```python
from build123d import *

# Parameters (mm, degrees)
BOSS_EXTRU_1_DEPTH           = 7.5
R_P_TITION_CIRCULAIRE1_COUNT = 33
ENL_V_MAT_EXTRU_3_DEPTH      = 129.364948487
ENL_V_MAT_EXTRU_3_DEPTH_BACK = 129.364948487
ESQUISSE7_R                  = 2.25


with BuildPart() as part:
    # Esquisse1 → Révolution1 (revolve)
    with BuildSketch(Plane.XY, mode=Mode.PRIVATE) as r_volution1_sk:
        Polygon((-63.3, 15), (-63.3, 0), (63.3, 0), (63.3, 15), (-35.8, 15), (-35.8, 12), (-43.3, 12), (-43.3, 15), align=None)
    revolve(r_volution1_sk.sketch.rotate(Axis((-63.3, 0, 0), (1, 0, 0)), 180), axis=Axis((-63.3, 0, 0), (1, 0, 0)))

    # Esquisse3 → Boss.-Extru.1 (add)
    with BuildSketch(Plane(origin=(-43.3, 0, 0), x_dir=(0, 0, -1), z_dir=(1, 0, 0))):
        Polygon((0.691111458, 13.454530338), (1.369204766, 11.251751142), (-0.629722527, 11.317246794), (0.191111458, 13.470913037), align=None)
    boss_extru_1 = extrude(amount=BOSS_EXTRU_1_DEPTH)

    # Répétition circulaire1: Boss.-Extru.1 ×33 about axis
    r_p_tition_circulaire1_axis = Axis((0, 0, 0), (1, 0, 0))
    for i in range(1, R_P_TITION_CIRCULAIRE1_COUNT):
        add(boss_extru_1.rotate(r_p_tition_circulaire1_axis, i * 360 / R_P_TITION_CIRCULAIRE1_COUNT))

    # Esquisse7 → Enlèv. mat.-Extru.3 (cut, two sides: drawn at the far end of the back side and taken through both)
    with BuildSketch(Plane.ZY.offset(63.3).offset(-ENL_V_MAT_EXTRU_3_DEPTH_BACK)):
        with Locations(Location((0, 0, 0), (0, 0, 90))):
            Circle(ESQUISSE7_R)
    extrude(amount=ENL_V_MAT_EXTRU_3_DEPTH + ENL_V_MAT_EXTRU_3_DEPTH_BACK, mode=Mode.SUBTRACT)


solid = part.part
```
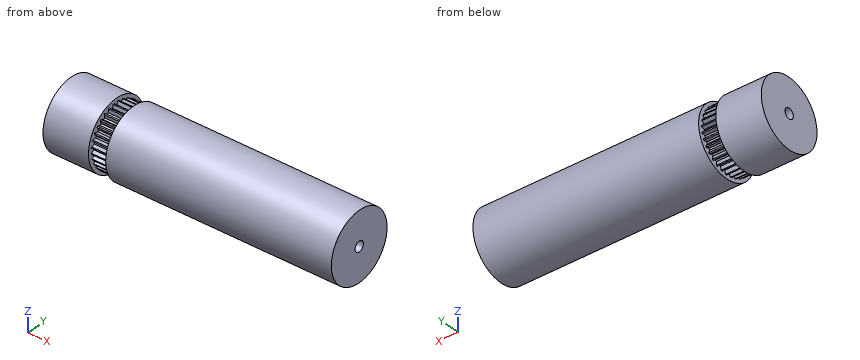
CAD build for the part. Positions are in the model's coordinates, mm. Round coordinates to 2 decimals unless told otherwise and drop trailing zeros. Write each loop counter-clockwise with the first axis right and the second up, starting at its lowest first coordinate (ties: lowest second). Pieces come first, ordered by that corner, then holes. Notation, with made-up numbers: (-37, 9) -> (-13, 9) arc R27 cw to (-13, 44) -> close; hole circle Ø8 at (61, 45). An arc over 180 degrees is marked (long way). Answer in a Markdown table with one row per item. Add a question column.
Item 1: Drill centre lines: line 1 (X direction, y = 10, z = 11); line 2 (Z direction, x = 27, y = 0); line 3 (Z direction, x = -36, y = 0). Where is each one in solid material? Low to high. Write a range as from..to.
Item 2: Saw through at A-A, the plane x = 5. Write the cut outline in (y, z).
Item 3: Drop flat-ended pins along their axis: pin 1 Ø12 at (x, z) = (31.5, -1.5) entering from +Y; pin 2 Ø1.5 at (x, y) = (13, 10) entering from -Z; pin 3 Ø3 at (x, y) = (-8.5, -10) entering from -Z; pin 4 Ø1.5 at (x, z) = (-28.5, 6.5) entering from +Y. Give the stop position or say it passes through.
Findings below:
| question | item | result |
|---|---|---|
| 1 | line 1 | x = -63.3..-43.3, -35.8..63.3 |
| 1 | line 2 | z = -15..-2.25, 2.25..15 |
| 1 | line 3 | z = -13.47..-2.25, 2.25..12 |
| 2 | outline | circle Ø30 at (0, 0); hole circle Ø4.5 at (0, 0) |
| 3 | pin 1 | stops at y = 15 |
| 3 | pin 2 | stops at z = -11.81 |
| 3 | pin 3 | stops at z = -12.36 |
| 3 | pin 4 | stops at y = 13.85 |
